Here's the drawing with two shaded views (mm, measured from the low corner). I have some questions. Give positions to 0.01 mm unless a question says otherwise; leave off trailing zeros. Use one line per item in the form item = value.
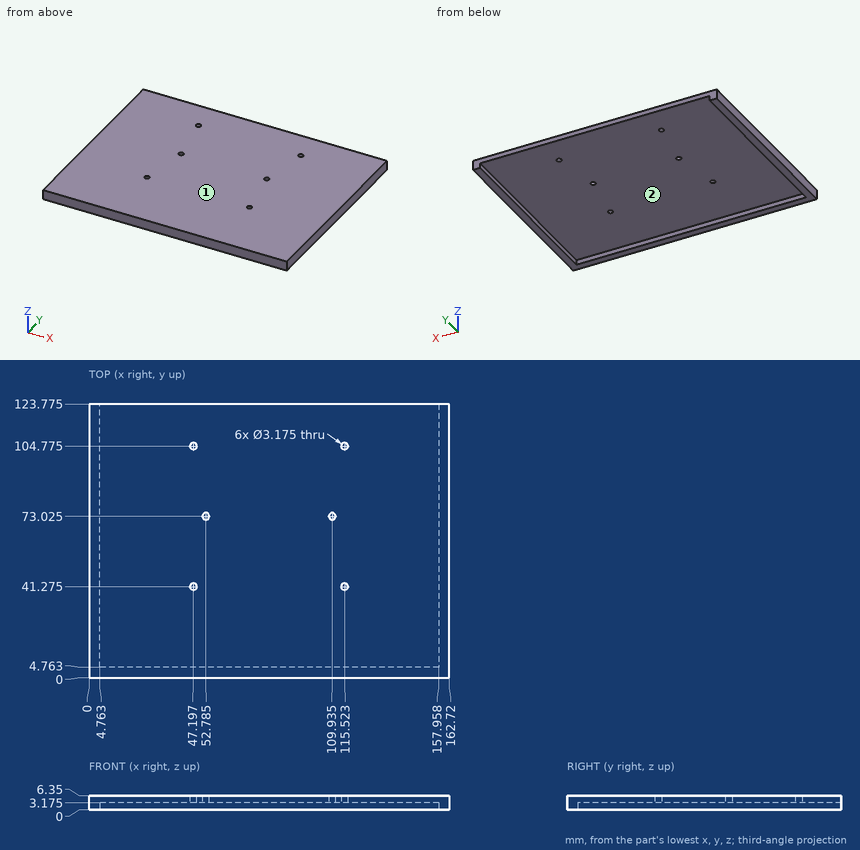
1. If we mould it in two halves opening along X, with no side actions, what happens to the marked faces 1 and 2? For each: pulls with the +X half, pulls with the -X half, needs draft (parallel to the pull), parting line crosses it, or undercut.
Response values:
face_1 = needs draft
face_2 = undercut
2. For pin 1 (1 mm diameter, centred on x = 80, z = 2, fed in from +Y); pin 2 (2.5 mm diameter, centred on x = 115.52, y = 41.28, fed in from -Z); pin 3 (3.5 mm diameter, centred on x = 109.94, y = 73.03, fed in from -Z) (1 decimal), each with a flat end and sliding along its axis, tell me the tip position at first contact or that it passes through.
Response values:
pin_1 = 4.76
pin_2 = through
pin_3 = 3.2
3. If I drill on line 1 (X direction, y = 27, z = 1.25); line 2 (Y direction, x = 82.5, z = 3), over which ranges is the centre line in solid material (lowest first)? Write a range as from..to.
Response values:
line_1 = 0..4.76, 157.96..162.72
line_2 = 0..4.76
